Here's how the part is built. I have some questions about the finished solid (model axes, mm). A direction names the side the tool comes from. Coordinates: 2 decimals unless noted, no trailing zeros. Loops run counter-clockwise (first coordinate to the right, second up) from the corner with the lowest first, then second, coordinate; pieces in that order, holes last.
```python
from build123d import *

# Parameters (mm, degrees)
SKETCH1_R           = 39
SKETCH1_R_2         = 1.55
SKETCH1_R_3         = 4
BOSS_EXTRUDE2_DEPTH = 6
SKETCH2_R           = 8
CUT_EXTRUDE1_DEPTH  = 3
SKETCH3_R           = 3.5
CUT_EXTRUDE2_DEPTH  = 4
SKETCH4_R           = 3.5
CUT_EXTRUDE3_DEPTH  = 3


with BuildPart() as part:
    # Sketch1 → Boss-Extrude2 (new body)
    with BuildSketch(Plane.XY):
        Circle(SKETCH1_R)
        with Locations((-27, 0)):
            Circle(SKETCH1_R_2, mode=Mode.SUBTRACT)
        with Locations((-19.091883092, 19.091883092)):
            Circle(SKETCH1_R_2, mode=Mode.SUBTRACT)
        with Locations((0, 27)):
            Circle(SKETCH1_R_2, mode=Mode.SUBTRACT)
        with Locations((19.091883092, 19.091883092)):
            Circle(SKETCH1_R_2, mode=Mode.SUBTRACT)
        with Locations((27, 0)):
            Circle(SKETCH1_R_2, mode=Mode.SUBTRACT)
        with Locations((19.091883092, -19.091883092)):
            Circle(SKETCH1_R_2, mode=Mode.SUBTRACT)
        with Locations((0, -27)):
            Circle(SKETCH1_R_2, mode=Mode.SUBTRACT)
        with Locations((-19.091883092, -19.091883092)):
            Circle(SKETCH1_R_2, mode=Mode.SUBTRACT)
        Circle(SKETCH1_R_3, mode=Mode.SUBTRACT)
        with Locations((-35, 0)):
            Circle(SKETCH1_R_2, mode=Mode.SUBTRACT)
        with Locations((-24.748737342, 24.748737342)):
            Circle(SKETCH1_R_2, mode=Mode.SUBTRACT)
        with Locations((0, 35)):
            Circle(SKETCH1_R_2, mode=Mode.SUBTRACT)
        with Locations((24.748737342, 24.748737342)):
            Circle(SKETCH1_R_2, mode=Mode.SUBTRACT)
        with Locations((35, 0)):
            Circle(SKETCH1_R_2, mode=Mode.SUBTRACT)
        with Locations((24.748737342, -24.748737342)):
            Circle(SKETCH1_R_2, mode=Mode.SUBTRACT)
        with Locations((0, -35)):
            Circle(SKETCH1_R_2, mode=Mode.SUBTRACT)
        with Locations((-24.748737342, -24.748737342)):
            Circle(SKETCH1_R_2, mode=Mode.SUBTRACT)
    extrude(amount=BOSS_EXTRUDE2_DEPTH)

    # Sketch2 → Cut-Extrude1 (cut)
    with BuildSketch(Plane.XY.offset(6)):
        Circle(SKETCH2_R)
    extrude(amount=-CUT_EXTRUDE1_DEPTH, mode=Mode.SUBTRACT)

    # Sketch3 → Cut-Extrude2 (cut)
    with BuildSketch(Plane(origin=(0, 0, 0), x_dir=(-1, 0, 0), z_dir=(0, 0, -1))):
        with Locations((0, 27)):
            Circle(SKETCH3_R)
        with Locations((19.091883092, 19.091883092)):
            Circle(SKETCH3_R)
        with Locations((27, 0)):
            Circle(SKETCH3_R)
        with Locations((19.091883092, -19.091883092)):
            Circle(SKETCH3_R)
        with Locations((0, -27)):
            Circle(SKETCH3_R)
        with Locations((-19.091883092, -19.091883092)):
            Circle(SKETCH3_R)
        with Locations((-27, 0)):
            Circle(SKETCH3_R)
        with Locations((-19.091883092, 19.091883092)):
            Circle(SKETCH3_R)
    extrude(amount=-CUT_EXTRUDE2_DEPTH, mode=Mode.SUBTRACT)

    # Sketch4 → Cut-Extrude3 (cut)
    with BuildSketch(Plane.XY.offset(6)):
        with Locations((-35, 0)):
            Circle(SKETCH4_R)
        with Locations((-24.748737342, 24.748737342)):
            Circle(SKETCH4_R)
        with Locations((0, 35)):
            Circle(SKETCH4_R)
        with Locations((24.748737342, 24.748737342)):
            Circle(SKETCH4_R)
        with Locations((35, 0)):
            Circle(SKETCH4_R)
        with Locations((24.748737342, -24.748737342)):
            Circle(SKETCH4_R)
        with Locations((0, -35)):
            Circle(SKETCH4_R)
        with Locations((-24.748737342, -24.748737342)):
            Circle(SKETCH4_R)
    extrude(amount=-CUT_EXTRUDE3_DEPTH, mode=Mode.SUBTRACT)


solid = part.part
```
1. On a 3-axis mill with a long thin cutter (end or side, diameter ignored), from which of +Z, -Z, +X, -X, +Y, -Y can I reach the whole of each face in a straight line? I mean faces 4 (the cylindrical face through (-0.46, -31.53, 4.52)), 5 (the cylindrical face through (-20.234, 20.139, 4.986)), 6 (the cylindrical face through (-18.3, -22.5, 2)). Say none if no direction works.
2. I want a section at D-D (x = 9.5). Please give me the cut outline in (y, z), then the cut area to 3 significant figures.
3. I want a section at B-B (z = 1.35). Give the number of separate pieces and of enclosed holes in the cut face, then the cut area to 3 significant figures.
4. For pin 1 (5.5 mm diameter, centred on x = 18, y = 18, fed in from -Z); pin 2 (8 mm diameter, centred on x = 2, y = 1.5, fed in from +Z); pin 3 (6.5 mm diameter, centred on x = 19.09, y = -19.09, fed in from -Z); pin 4 (1.9 mm diameter, centred on x = 0, y = 27, fed in from -Z), each with a flat end and sliding along its axis, tell me the tip position at first contact or that it passes through.
5. We'd pull the mould along Y, two halves only. Please class faces 1 (the flat face through (8, -8, 6)), 2 (the cylindrical face through (-5.077, 38.668, 2.958)), 3 (the flat face through (-23, 24, 3)): +Y half, -Y half, draft (parallel to the pull), parting line (faces both ways), or undercut.
6. I need wall thicknesses on line 1 along Y through (x, z) = (0, 5.35); line 2 along Y through (x, z) = (19, 4.4); line 3 along Y through (x, z) = (17, 2.5). Which ranges of each line are inside material? Lowest first, please.
7. I want a section at A-A (x = 35). Please give me the cut outline in (y, z), then the cut area to 3 significant figures.
Response values:
1. face 4: +Z
1. face 5: +Z, -Z
1. face 6: -Z
2. outline: (-37.83, 0) - (37.83, 0) - (37.83, 6) - (-37.83, 6) - close
2. area: 454 mm2
3. separate pieces: 1
3. enclosed holes: 17
3. area: 4,360 mm2
4. pin 1: stops at z = 0
4. pin 2: stops at z = 3
4. pin 3: stops at z = 4
4. pin 4: passes through
5. face 1: draft
5. face 2: parting line
5. face 3: undercut
6. line 1: y = -39 to -38.5, -31.5 to -28.55, -25.45 to -8, 8 to 25.45, 28.55 to 31.5, 38.5 to 39
6. line 2: y = -34.06 to -20.64, -17.54 to 17.54, 20.64 to 34.06
6. line 3: y = -35.1 to -21.9, -16.29 to 16.29, 21.9 to 35.1
7. outline: (-17.2, 0) - (-1.55, 0) - (-1.55, 3) - (-3.5, 3) - (-3.5, 6) - (-17.2, 6) - close; (1.55, 0) - (17.2, 0) - (17.2, 6) - (3.5, 6) - (3.5, 3) - (1.55, 3) - close
7. area: 176 mm2
